Geometry check sheet. Reference: the model listing, model coordinates, mm. Give positions to 0.01 mm unless a question says otherwise; leave off trailing zeros. Loops run counter-clockwise (first coordinate to the right, second up) from the corner with the lowest first, then second, coordinate; pieces in that order, holes last. Notation, with made-up numbers: (4.25, -32.5) -> (8.25, -32.5) arc R21 cw to (8.25, -12.5) -> close; hole circle Ø6 at (-29, -10.5). An arc over 180 degrees is marked (long way). One line per question, with ' | ' between items.
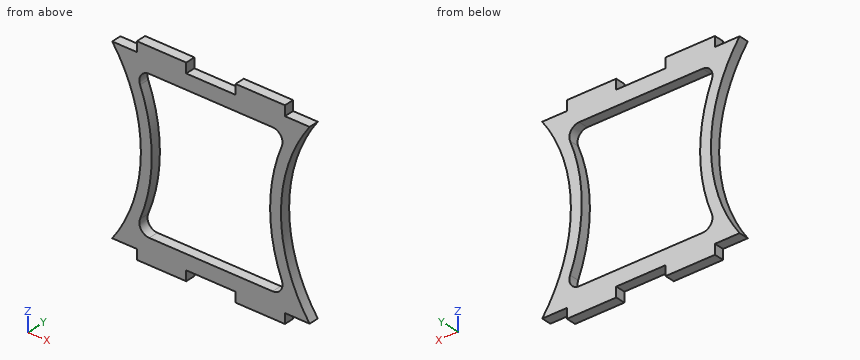
from build123d import *

# Parameters (mm, degrees)
BOSS_EXTRUDE1_DEPTH = 2


with BuildPart() as part:
    # Sketch1 → Boss-Extrude1 (new body)
    with BuildSketch(Plane(origin=(0, 0, 0), x_dir=(1, 0, 0), z_dir=(0, 1, 0))):
        with BuildLine():
            Line((-20, -18), (-15, -18))
            Line((-15, -18), (-15, -20))
            Line((-15, -20), (-5, -20))
            Line((-5, -20), (-5, -18))
            Line((-5, -18), (5, -18))
            Line((5, -18), (5, -20))
            Line((5, -20), (15, -20))
            Line((15, -20), (15, -18))
            Line((15, -18), (20, -18))
            ThreePointArc((20, -18), (14.194156399, 0), (20, 18))
            Line((20, 18), (15, 18))
            Line((15, 18), (15, 20))
            Line((15, 20), (5, 20))
            Line((5, 20), (5, 18))
            Line((5, 18), (-5, 18))
            Line((-5, 18), (-5, 20))
            Line((-5, 20), (-15, 20))
            Line((-15, 20), (-15, 18))
            Line((-15, 18), (-20, 18))
            ThreePointArc((-20, 18), (-14.194156399, 0), (-20, -18))
        make_face()
        with BuildLine():
            Line((-12.503846381, 15), (12.503846381, 15))
            ThreePointArc((12.503846381, 15), (14.160003724, 14.121223821), (14.360769445, 12.257142857))
            ThreePointArc((14.360769445, 12.257142857), (12, 0), (14.360769445, -12.257142857))
            ThreePointArc((14.360769445, -12.257142857), (14.160003724, -14.121223821), (12.503846381, -15))
            Line((12.503846381, -15), (-12.503846381, -15))
            ThreePointArc((-12.503846381, -15), (-14.160003724, -14.121223821), (-14.360769445, -12.257142857))
            ThreePointArc((-14.360769445, -12.257142857), (-12, 0), (-14.360769445, 12.257142857))
            ThreePointArc((-14.360769445, 12.257142857), (-14.160003724, 14.121223821), (-12.503846381, 15))
        make_face(mode=Mode.SUBTRACT)
    extrude(amount=BOSS_EXTRUDE1_DEPTH)


solid = part.part
Item 1: Scan lines: probe 1 along Z at (x, y) = (-4.5, 1.95); probe 2 along Z at (x, y) = (8, 1.75); probe 3 along X at (y, z) = (1.85, 10.5). Record each from-to range of solid material in increasing order.
Result:
probe 1: -18 to -15, 15 to 18 | probe 2: -20 to -15, 15 to 20 | probe 3: -16.04 to -13.72, 13.72 to 16.04
Item 2: Sectioned sample at B-B (y = 0.85). Record the cut outline in (x, z), plus the area to 3 significant figures.
Result:
outline: (-20, -18) -> (-15, -18) -> (-15, -20) -> (-5, -20) -> (-5, -18) -> (5, -18) -> (5, -20) -> (15, -20) -> (15, -18) -> (20, -18) arc R30.81 cw to (20, 18) -> (15, 18) -> (15, 20) -> (5, 20) -> (5, 18) -> (-5, 18) -> (-5, 20) -> (-15, 20) -> (-15, 18) -> (-20, 18) arc R30.81 cw to start; hole (-14.36, -12.26) arc R2 ccw to (-12.5, -15) -> (12.5, -15) arc R2 ccw to (14.36, -12.26) arc R33 cw to (14.36, 12.26) arc R2 ccw to (12.5, 15) -> (-12.5, 15) arc R2 ccw to (-14.36, 12.26) arc R33 cw to start | area: 454 mm2
Item 3: Sectioned sample at C-C (z = 13). Record the cut outline in (x, y).
Result:
outline: (-17.07, 0) -> (-14.5, 0) -> (-14.5, 2) -> (-17.07, 2) -> close; (14.5, 0) -> (17.07, 0) -> (17.07, 2) -> (14.5, 2) -> close
Item 4: Depth check by flat-ended pin: pin 1 Ø1 at (y, z) = (1.5, 19) entering from -X; pin 2 Ø0.6 at (y, z) = (0.5, 19) entering from +X; pin 3 Ø0.6 at (x, y) = (18.5, 1) entering from +Z. Enter the tip coordinate at first touch or a pass-through.
Result:
pin 1: x = -15 | pin 2: x = 15 | pin 3: z = 18
Item 5: Sectioned sample at A-A (x = 8). Record the cut outline in (y, z).
Result:
outline: (0, -20) -> (2, -20) -> (2, -15) -> (0, -15) -> close; (0, 15) -> (2, 15) -> (2, 20) -> (0, 20) -> close
Item 6: Sectioned sample at D-D (x = -13.5). Record the cut outline in (y, z).
Result:
outline: (0, -20) -> (2, -20) -> (2, -14.73) -> (0, -14.73) -> close; (0, -9.84) -> (2, -9.84) -> (2, 9.84) -> (0, 9.84) -> close; (0, 14.73) -> (2, 14.73) -> (2, 20) -> (0, 20) -> close
